Check sheet for the modelled part. Datum: model origin and axes. Units: mm. Face numbers are marked on the shaded views. A direction names the side the tool comes from. Round coordinates to 2 decimals unless told otherwise and drop trailing zeros. Order: outer loops, then holes, each group sorted by start corner. A loop starts at its lowest first (then second) coordinate and runs counter-clockwise, first axis right, second up.
Q1. Cross-section at A-A on z = 72.5. Record the cut outline in (x, y) (3 decimals).
Q2. Depth check by flat-ended pin: P1, Ø4.5, axis at x = 228.6, z = 109.9, coming from the -Y side (1 decimal); P2, Ø6.5, axis at x = 228.6, z = 21, coming from the +Y side; P3, Ø2, axis at x = -214.5, y = 29.5, coming from the -Z side. Enter the tip coordinate at first touch or a pass-through.
Q3. Cross-section at C-C on x = 85. Record the cut outline in (y, z).
Q4. Set-up check for the marked faces 1 and 2: record each of +Z, -Z, +X, -X, +Y, -Y from which the full face is reachable in a straight line by a thin tool's end or side.
Q5. Cross-section at B-B on x = 186. Record the cut outline in (y, z).
Q6. Scan lines: probe 1 along Y at (x, z) = (37.5, 76); probe 2 along Z at (x, y) = (50.8, 0.75). Record each from-to range of solid material in increasing order.
from build123d import *

# Parameters (mm, degrees)
SKETCH1_W             = 539.75
SKETCH1_H             = 127
BASE_FLANGE1_DEPTH    = 2.54
EDGE_FLANGE1_START    = -269.875
EDGE_FLANGE1_DEPTH    = 539.75
EDGE_FLANGE1_2_DEPTH  = 539.75
EDGE_FLANGE1_START_2  = -108.715226281
EDGE_FLANGE1_3_DEPTH  = 2.54
F_8_CLEARANCE_HOLE1_D = 4.9149
CUT_EXTRUDE1_DEPTH    = 335.555040238
DELETEFACE1_START     = -76.607285952
DELETEFACE1_OUTLINE_W = 2.54
DELETEFACE1_OUTLINE_H = 31
DELETEFACE1_DEPTH     = 85.478449448
FILLET1_R             = 6.35
F_8_CLEARANCE_HOLE2_D = 4.9149
SKETCH19_R            = 12.7
CUT_EXTRUDE2_DEPTH    = 335.555040319


with BuildPart() as part:
    # Base-Flange1: sheet metal written as solids
    # Sketch1 → Base-Flange1 (new body)
    with BuildSketch(Plane(origin=(0, 0, 0), x_dir=(1, 0, 0), z_dir=(0, 1, 0))):
        with Locations((0, -63.5)):
            Rectangle(SKETCH1_W, SKETCH1_H)
    extrude(amount=BASE_FLANGE1_DEPTH)

    # Edge-Flange1: read off the stored shape, not the designer's step
    # Edge-Flange1 outline → Edge-Flange1 (cut)
    with BuildSketch(Plane.YZ.offset(EDGE_FLANGE1_START)):
        with BuildLine():
            ThreePointArc((0, 123.641784424), (0.438981162, 125.280084424), (1.6383, 126.479403262))
            Line((1.6383, 126.479403262), (2.54, 127))
            Line((2.54, 127), (0, 127))
            Line((0, 127), (0, 123.641784424))
        make_face()
    extrude(amount=EDGE_FLANGE1_DEPTH, mode=Mode.SUBTRACT)

    # Edge-Flange1 2 outline → Edge-Flange1 2 (add)
    with BuildSketch(Plane.YZ.offset(EDGE_FLANGE1_START)):
        with BuildLine():
            Line((89.258181024, 177.066765158), (2.54, 127))
            Line((2.54, 127), (2.54, 123.641784424))
            ThreePointArc((2.54, 123.641784424), (2.638685688, 124.010084424), (2.9083, 124.279698737))
            Line((2.9083, 124.279698737), (90.528181024, 174.867060633))
            Line((90.528181024, 174.867060633), (89.258181024, 177.066765158))
        make_face()
    extrude(amount=EDGE_FLANGE1_2_DEPTH)

    # Edge-Flange1 3 outline → Edge-Flange1 3 (cut)
    with BuildSketch(Plane(origin=(0, 0, 0), x_dir=(1, 0, 0), z_dir=(0, 0.50000000000001, -0.8660254037844329)).offset(EDGE_FLANGE1_START_2)):
        with BuildLine():
            Line((-238.125, -165.833234842), (238.125, -165.833234842))
            ThreePointArc((238.125, -165.833234842), (225.935445104, -132.820002209), (195.216593352, -115.649943256))
            Line((195.216593352, -115.649943256), (59.186950142, -94.25854795))
            ThreePointArc((59.186950142, -94.25854795), (0, -89.633234842), (-59.186950142, -94.25854795))
            Line((-59.186950142, -94.25854795), (-195.216593352, -115.649943256))
            ThreePointArc((-195.216593352, -115.649943256), (-225.935445104, -132.820002209), (-238.125, -165.833234842))
        make_face()
    extrude(amount=EDGE_FLANGE1_3_DEPTH, mode=Mode.SUBTRACT)

    # #8 Clearance Hole1 (through all)
    with Locations(Plane(origin=(0, 0, 0), x_dir=(-1, 0, 0), z_dir=(0, -1, 0))):
        with Locations((-101.6, -20.995817153), (-127, -20.995817153), (-152.4, -20.995817153), (-177.8, -20.995817153), (-203.2, -20.995817153), (-228.6, -20.995817153), (152.4, -20.995817153), (177.8, -20.995817153), (203.2, -20.995817153), (228.6, -20.995817153), (-228.6, -109.895817153), (-203.2, -109.895817153), (-177.8, -109.895817153), (-152.4, -109.895817153), (-127, -109.895817153), (-101.6, -109.895817153), (-76.2, -109.895817153), (-50.8, -109.895817153), (-25.4, -109.895817153), (50.8, -109.895817153), (76.2, -109.895817153), (101.6, -109.895817153), (127, -109.895817153), (25.4, -109.895817153), (0, -109.895817153), (152.4, -109.895817153), (177.8, -109.895817153), (203.2, -109.895817153), (228.6, -109.895817153), (-254, -109.895817153), (-254, -59.095817153), (-254, -33.695817153), (-254, -8.295817153), (-254, -84.495817153), (254, -109.895817153), (254, -84.495817153), (254, -59.095817153), (254, -33.695817153), (254, -8.295817153), (254, -20.995817153), (-254, -20.995817153)):
            Hole(F_8_CLEARANCE_HOLE1_D / 2)

    # Sketch12 → Cut-Extrude1 (cut, through all)
    with BuildSketch(Plane(origin=(0, 2.54, 0), x_dir=(1, 0, 0), z_dir=(0, 1, 0))):
        with BuildLine():
            Line((10.750764667, -35.632627255), (10.064214119, -22.532462404))
            ThreePointArc((10.064214119, -22.532462404), (8.049198612, -18.216593523), (3.600048039, -16.515984552))
            ThreePointArc((3.600048039, -16.515984552), (-48.154577437, -10.211146763), (-96.127816756, 10.206016283))
            ThreePointArc((-96.127816756, 10.206016283), (-100.831198663, 10.957820999), (-104.734187721, 8.227676662))
            Line((-104.734187721, 8.227676662), (-111.878840363, -2.77412362))
            ThreePointArc((-111.878840363, -2.77412362), (-117.278135386, -46.313585823), (-86.367734849, -77.4485227))
            ThreePointArc((-86.367734849, -77.4485227), (-67.71223858, -83.201331827), (-48.679700327, -87.547001114))
            ThreePointArc((-48.679700327, -87.547001114), (-6.343039783, -76.038555102), (10.750764667, -35.632627255))
        make_face()
    extrude(amount=-CUT_EXTRUDE1_DEPTH, mode=Mode.SUBTRACT)

    # DeleteFace1: read off the stored shape, not the designer's step
    # DeleteFace1 outline → DeleteFace1 (cut)
    with BuildSketch(Plane(origin=(0, 0, 0), x_dir=(0, 1, 0), z_dir=(0.9986295347545738, 0, -0.052335956242945486)).offset(DELETEFACE1_START)):
        with Locations((1.27, 9.5)):
            Rectangle(DELETEFACE1_OUTLINE_W, DELETEFACE1_OUTLINE_H)
    extrude(amount=DELETEFACE1_DEPTH, mode=Mode.SUBTRACT)

    # Fillet1
    fillet1_edges = [part.edges().sort_by_distance(p)[0] for p in [
        (8.883337802, 1.27, 0),
        (-110.07730342, 1.27, 0),
    ]]
    fillet(fillet1_edges, radius=FILLET1_R)

    # #8 Clearance Hole2 (through all)
    with Locations(Plane(origin=(0, -53.08761314, 91.950443212), x_dir=(-1, 0, 0), z_dir=(0, 0.5000000000000102, -0.8660254037844328))):
        with Locations((-254, 144.334416739), (-254, 118.934416739), (-254, 93.534416739), (254, 93.534416739), (254, 118.934416739), (254, 144.334416739)):
            Hole(F_8_CLEARANCE_HOLE2_D / 2)

    # Sketch19 → Cut-Extrude2 (cut, through all)
    with BuildSketch(Plane(origin=(0, 2.54, 0), x_dir=(1, 0, 0), z_dir=(0, 1, 0))):
        with Locations(Location((152.4, -65.445817153, 0), (0, 0, 270))):
            Circle(SKETCH19_R)
        with Locations(Location((-152.4, -65.445817153, 0), (0, 0, 270))):
            Circle(SKETCH19_R)
    extrude(amount=-CUT_EXTRUDE2_DEPTH, mode=Mode.SUBTRACT)


solid = part.part
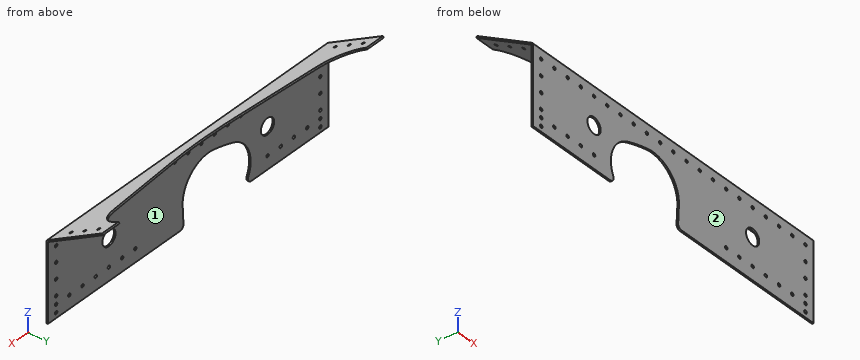
Results found:
1. outline: (-269.875, 0) - (-162.961, 0) - (-162.961, 2.54) - (-269.875, 2.54) - close; (-141.839, 0) - (-96.61, 0) - (-96.61, 2.54) - (-141.839, 2.54) - close; (-2.685, 0) - (141.839, 0) - (141.839, 2.54) - (-2.685, 2.54) - close; (162.961, 0) - (269.875, 0) - (269.875, 2.54) - (162.961, 2.54) - close
2. P1: passes through
2. P2: stops at y = 2.54
2. P3: stops at z = 139.06
3. outline: (0, 0) - (2.54, 0) - (2.54, 123.64) arc R0.74 cw to (2.91, 124.28) - (32.06, 141.11) - (30.79, 143.31) - (1.64, 126.48) arc R3.28 ccw to (0, 123.64) - close
4. face 1: -Z, +X, -X, +Y
4. face 2: +Z, -Z, +X, -X, -Y
5. outline: (0, 0) - (2.54, 0) - (2.54, 123.64) arc R0.74 cw to (2.91, 124.28) - (45.81, 149.05) - (44.54, 151.25) - (1.64, 126.48) arc R3.28 ccw to (0, 123.64) - close
6. probe 1: y = 0 to 2.54
6. probe 2: z = 0 to 107.44, 112.35 to 125.73
